```python
from build123d import *

# Parameters (mm, degrees)
F0_R     = 6.35
F1_DEPTH = 12.7
F2_W     = 12.7
F2_H     = 25.4
F3_DEPTH = 25.4
F4_W     = 25.4
F4_H     = 6.35
F5_DEPTH = 12.7
F7_DEPTH = 25.4
F9_DEPTH = 25.4


with BuildPart() as f1:
    # F0 (on Top) → F1 (new body)
    with BuildSketch(Plane.XY):
        with BuildLine():
            Line((0, 25.4), (0, 0))
            Line((0, 0), (44.45, 0))
            ThreePointArc((44.45, 0), (57.15, 12.7), (44.45, 25.4))
            Line((44.45, 25.4), (0, 25.4))
        make_face()
        with Locations((25.4, 12.7)):
            Circle(F0_R, mode=Mode.SUBTRACT)
        with Locations((44.45, 12.7)):
            Circle(F0_R, mode=Mode.SUBTRACT)
    extrude(amount=F1_DEPTH)

    # F2 (on face) → F3 (join)
    with BuildSketch(Plane.XZ):
        with Locations((6.35, 25.4)):
            Rectangle(F2_W, F2_H)
    extrude(amount=-F3_DEPTH)

    # F4 (on face) → F5 (join)
    with BuildSketch(Plane.YZ.offset(12.7)):
        with Locations((12.7, 41.275)):
            Rectangle(F4_W, F4_H)
    extrude(amount=-F5_DEPTH)

    # F6 (on face) → F7 (cut)
    with BuildSketch(Plane.YZ.offset(12.7)):
        with BuildLine():
            ThreePointArc((15.8657383942, 44.45), (21.2446497119, 42.1935630666), (25.4, 38.1))
            Line((25.4, 38.1), (25.4, 44.45))
            Line((25.4, 44.45), (15.8657383942, 44.45))
        make_face()
        with BuildLine():
            ThreePointArc((0, 38.1), (4.1553502881, 42.1935630666), (9.5342616058, 44.45))
            Line((9.5342616058, 44.45), (0, 44.45))
            Line((0, 44.45), (0, 38.1))
        make_face()
    extrude(amount=-F7_DEPTH, mode=Mode.SUBTRACT)

    # F8 (on face) → F9 (cut)
    with BuildSketch(Plane.YZ.offset(12.7)):
        with BuildLine():
            ThreePointArc((9.5342616058, 44.45), (7.9137921468, 44.0166926131), (6.35, 43.4098724745))
            Line((6.35, 43.4098724745), (6.35, 30.7098724745))
            ThreePointArc((6.35, 30.7098724745), (12.7, 24.3598724745), (19.05, 30.7098724745))
            Line((19.05, 30.7098724745), (19.05, 43.4098724745))
            ThreePointArc((19.05, 43.4098724745), (17.4862078532, 44.0166926131), (15.8657383942, 44.45))
            Line((15.8657383942, 44.45), (9.5342616058, 44.45))
        make_face()
    extrude(amount=-F9_DEPTH, mode=Mode.SUBTRACT)


solid = f1.part
```
Work out the finished part from the listing and answer in its coordinate system (mm). A direction names the side the tool comes from. Give positions to 0.01 mm unless a question says otherwise; leave off trailing zeros. Loops run counter-clockwise (first coordinate to the right, second up) from the corner with the lowest first, then second, coordinate; pieces in that order, holes last. Notation, with made-up numbers: M -1.5,-2 L 27.5,-2 A23 cw 27.5,11 Z; hole C 63.25,24 d6. An arc over 180 degrees is marked long. One line per item, written item: value. Start each with the question number.
1. Determine the mould class of faces 4 (the face through (28, 19, 0)), 5 (the face through (6, 19.05, 37)), 6 (the face through (6.44, 22.54, 41.23)) for opening direction Y: released by +Y, released by -Y, zero draft, split by the parting line, or undercut.
2. Find section D-D (x = 11). Give the vertices of the cut face in (y, z).
3. Find section B-B (y = 12.7). Give the vertices of the cut face in (x, z), and give its area (3 significant figures).
4. Which of the six approach directions +Z, -Z, +X, -X, +Y, -Y give full straight-line access (tool end or side, diameter ignored) to faces 1 (the face through (18, 0, 10)), 2 (the face through (12.7, 9.7, 24.9)), 3 (the face through (6, 6.35, 37))?
5. Find section C-C (z = 10). Give the vertices of the cut face in (x, y), and give its area (3 significant figures).
6. Find the intervals of material crossed by probe 1 along Y at (x, z) = (7, 35); probe 2 along Y at (x, z) = (25, 3); probe 3 along Z at (x, y) = (55, 10), in increasing order.
7. Find section A-A (x = 25.4). Give the vertices of the cut face in (y, z), and give its area (3 significant figures).
8. Each of these flat-tipped pins is pushed along its axis until it touches: P1, Ø3, axis at y = 3.5, z = 37, coming from the +X side; P2, Ø1, axis at x = 37, y = 17, coming from the +Z side. Where does it stop, or does it pass through?
Reported:
1. face 4: zero draft
1. face 5: undercut
1. face 6: released by +Y
2. outline: M 0,0 L 25.4,0 L 25.4,38.1 A15.41 ccw 19.05,43.41 L 19.05,30.71 A6.35 cw 6.35,30.71 L 6.35,43.41 A15.41 ccw 0,38.1 Z
3. outline: M 0,0 L 19.05,0 L 19.05,12.7 L 12.7,12.7 L 12.7,24.36 L 0,24.36 Z; M 31.75,0 L 38.1,0 L 38.1,12.7 L 31.75,12.7 Z; M 50.8,0 L 57.15,0 L 57.15,12.7 L 50.8,12.7 Z
3. area: 551 mm²
4. face 1: +Z, -Z, +X, -X, -Y
4. face 2: +Z, +X, +Y, -Y
4. face 3: +Z, +X, -X
5. outline: M 0,0 L 44.45,0 A12.7 ccw 44.45,25.4 L 0,25.4 Z; hole C 25.4,12.7 d12.7; hole C 44.45,12.7 d12.7
5. area: 1,130 mm²
6. probe 1: y = 0 to 6.35, 19.05 to 25.4
6. probe 2: y = 0 to 6.36, 19.04 to 25.4
6. probe 3: z = 0 to 12.7
7. outline: M 0,0 L 6.35,0 L 6.35,12.7 L 0,12.7 Z; M 19.05,0 L 25.4,0 L 25.4,12.7 L 19.05,12.7 Z
7. area: 161 mm²
8. P1: stops at x = 12.7
8. P2: stops at z = 12.7
